Check sheet for the drawn part. Datum: minimum x, y, z corner. Units: mm. Round coordinates to 2 decimals unless told otherwise and drop trailing zeros. Write each loop counter-clockwise with the first axis right and the second up, starting at its lowest first coordinate (ties: lowest second). Pieces come first, ordered by that corner, then holes. Notation, with made-up numbers: M -21,89.5 L 9,89.5 A16 cw 9,118.5 Z; hole C -26,36 d7. An arc over 180 degrees is marked long. One line per item, written item: value. Start each with the question number.
1. Scan lines: probe 1 along Y at (x, z) = (9.75, 0.65); probe 2 along X at (y, z) = (10.25, 0.85); probe 3 along X at (y, z) = (8.75, 0.65). Record each from-to range of solid material in increasing order. Write a range as [from, to].
2. Section check B-B (y = 12.5). Record the boundary of the cut face in (x, z), and give its area (3 significant figures).
3. Section check C-C (z = 0.7). Record the boundary of the cut face in (x, y).
4. Section check A-A (x = 9.75). Record the boundary of the cut face in (y, z).
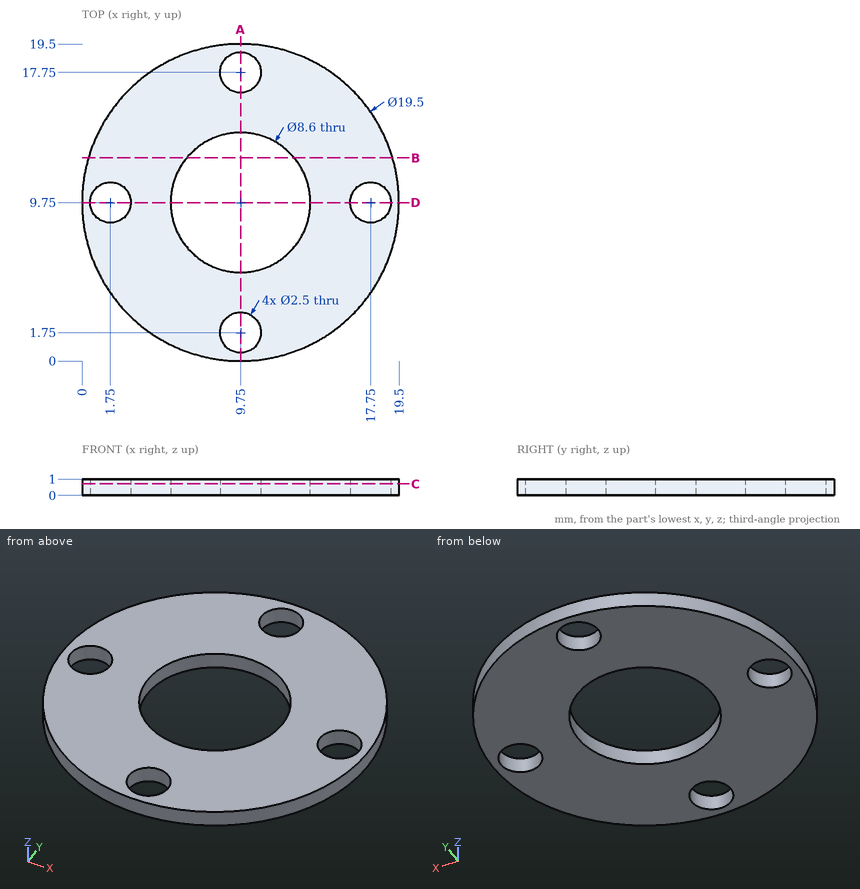
Result sheet:
1. probe 1: y = [0, 0.5], [3, 5.45], [14.05, 16.5], [19, 19.5]
1. probe 2: x = [0.01, 0.6], [2.9, 5.48], [14.02, 16.6], [18.9, 19.49]
1. probe 3: x = [0.05, 1], [2.5, 5.57], [13.93, 17], [18.5, 19.45]
2. outline: M 0.4,0 L 6.44,0 L 6.44,1 L 0.4,1 Z; M 13.06,0 L 19.1,0 L 19.1,1 L 13.06,1 Z
2. area: 12.1 mm2
3. outline: C 9.75,9.75 d19.5; hole C 1.75,9.75 d2.5; hole C 9.75,9.75 d8.6; hole C 9.75,1.75 d2.5; hole C 9.75,17.75 d2.5; hole C 17.75,9.75 d2.5
4. outline: M 0,0 L 0.5,0 L 0.5,1 L 0,1 Z; M 3,0 L 5.45,0 L 5.45,1 L 3,1 Z; M 14.05,0 L 16.5,0 L 16.5,1 L 14.05,1 Z; M 19,0 L 19.5,0 L 19.5,1 L 19,1 Z
